Answer from the drawing. Dimensions are ordinates in mm from the lowest x, y and z of the part. Coordinates: 2 decimals unless noted, no trailing zeros. Order: outer loops, then holes, each group sorted by start corner. A loop starts at its lowest first (then second) coordinate and runs counter-clockwise, first axis right, second up. Notation, with made-up numbers: (25, 46.25) - (36, 46.25) arc R30 cw to (36, 76.25) - close; hole circle Ø6 at (78.25, 60). An arc over 180 degrees is marked (long way). Answer as a JSON object with one key per item and string values. Group by question number.
1) Each of these flat-tipped pins is pushed along its axis until it touches: P1, Ø3, axis at x = 17, z = 74.5, coming from the +Y side (1 decimal); P2, Ø12, axis at x = 20, z = 144.5, coming from the -Y side; P3, Ø3, axis at x = 20.5, y = 21.5, coming from the +Z side. Where does it stop, or does it pass through?
2) Find the intervals of material crossed by line 1 along Y through (x, z) = (11.5, 10.5); line 2 along Y through (x, z) = (3.75, 85) (1 decimal); line 3 along Z through (x, y) = (10, 2) (1 decimal), in increasing order.
3) Section B-B (z = 170.5) is taken. Give the vertices of the cut face in (x, y), plus the area to 3 significant figures.
4) Section A-A (y = 12.5) is taken. Give the vertices of the cut face in (x, z), plus the area to 3 significant figures.
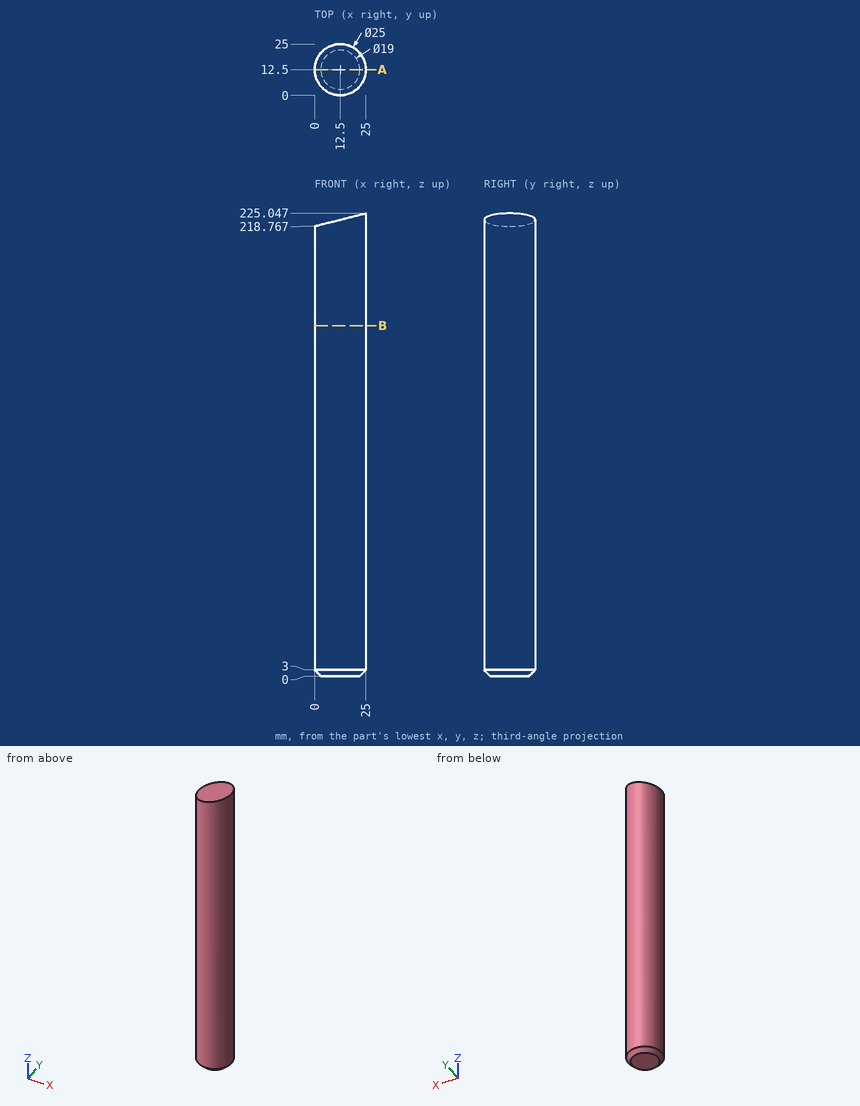
Report:
{
 "1": {"P1": "stops at y = 24.6", "P2": "stops at y = 0.09", "P3": "stops at z = 224.25"},
 "2": {"line 1": "y = 0.04 to 24.96", "line 2": "y = 3.6 to 21.4", "line 3": "z = 1.3 to 221.3"},
 "3": {"outline": "circle Ø25 at (12.5, 12.5)", "area": "491 mm²"},
 "4": {"outline": "(0, 3) - (3, 0) - (22, 0) - (25, 3) - (25, 225.05) - (0, 218.77) - close", "area": "5,540 mm²"}
}
